from build123d import *

# Parameters (mm, degrees)
SKETCH1_W           = 57.02
SKETCH1_H           = 36.2
SKETCH1_R           = 2.2
BOSS_EXTRUDE1_DEPTH = 4
SKETCH2_W           = 57.02
SKETCH2_H           = 4
BOSS_EXTRUDE2_DEPTH = 29.05
SKETCH3_W           = 4
SKETCH3_H           = 42.02
BOSS_EXTRUDE3_DEPTH = 26
SKETCH5_R           = 7
CUT_EXTRUDE1_DEPTH  = 4
SKETCH6_W           = 42.02
SKETCH6_H           = 30
BOSS_EXTRUDE4_DEPTH = 2.5
SKETCH7_W           = 16
SKETCH7_H           = 16
CUT_EXTRUDE2_DEPTH  = 6.5


with BuildPart() as part:
    # Sketch1 → Boss-Extrude1 (new body)
    with BuildSketch(Plane(origin=(0, 0, 0), x_dir=(0, 0, -1), z_dir=(1, 0, 0))):
        Rectangle(SKETCH1_W, SKETCH1_H)
        with Locations((-24.51, -4.25)):
            Circle(SKETCH1_R, mode=Mode.SUBTRACT)
        with Locations((-24.51, -14.1)):
            Circle(SKETCH1_R, mode=Mode.SUBTRACT)
        with Locations((24.51, -4.25)):
            Circle(SKETCH1_R, mode=Mode.SUBTRACT)
        with Locations((24.51, -14.1)):
            Circle(SKETCH1_R, mode=Mode.SUBTRACT)
    extrude(amount=BOSS_EXTRUDE1_DEPTH)

    # Sketch2 → Boss-Extrude2 (add)
    with BuildSketch(Plane(origin=(4, 0, 0), x_dir=(0, 0, -1), z_dir=(1, 0, 0))):
        with Locations((0, 16.1)):
            Rectangle(SKETCH2_W, SKETCH2_H)
    extrude(amount=BOSS_EXTRUDE2_DEPTH)

    # Sketch3 → Boss-Extrude3 (add)
    with BuildSketch(Plane.XZ.offset(-14.1)):
        with Locations((31.05, 7.5)):
            Rectangle(SKETCH3_W, SKETCH3_H)
    extrude(amount=BOSS_EXTRUDE3_DEPTH)

    # Sketch5 → Cut-Extrude1 (cut)
    with BuildSketch(Plane(origin=(0, 18.1, 0), x_dir=(1, 0, 0), z_dir=(0, 1, 0))):
        with Locations((19, -10.79)):
            Circle(SKETCH5_R)
    extrude(amount=-CUT_EXTRUDE1_DEPTH, mode=Mode.SUBTRACT)

    # Sketch6 → Boss-Extrude4 (add)
    with BuildSketch(Plane(origin=(33.05, 0, 0), x_dir=(0, 0, -1), z_dir=(1, 0, 0))):
        with Locations((-7.5, 3.1)):
            Rectangle(SKETCH6_W, SKETCH6_H)
    extrude(amount=BOSS_EXTRUDE4_DEPTH)

    # Sketch7 → Cut-Extrude2 (cut)
    with BuildSketch(Plane(origin=(35.55, 0, 0), x_dir=(0, 0, -1), z_dir=(1, 0, 0))):
        with Locations((-7.51, 8.1)):
            Rectangle(SKETCH7_W, SKETCH7_H)
    extrude(amount=-CUT_EXTRUDE2_DEPTH, mode=Mode.SUBTRACT)


solid = part.part
For this review, take the finished solid that the model builds, in its own axes (mm). A direction names the side the tool comes from. Round coordinates to 2 decimals unless told otherwise and drop trailing zeros. Write each loop counter-clockwise with the first axis right and the second up, starting at its lowest first coordinate (ties: lowest second). Pieces come first, ordered by that corner, then holes. Notation, with made-up numbers: (-31.75, -36) -> (12.25, -36) arc R12 cw to (12.25, -13) -> close; hole circle Ø5 at (-17, 88.5). An arc over 180 degrees is marked (long way). Put each result on its own line as item: value.
Q1. Clearance check with flat-ended pins moving along their axes: pin 1 Ø1.5 at (y, z) = (1, -17.5) entering from +X; pin 2 Ø3 at (x, z) = (32, 9.5) entering from -Y; pin 3 Ø1 at (x, y) = (29.5, 5.5) entering from -Z; pin 4 Ø8.5 at (x, z) = (19, 8.5) entering from -Y. State where each tip first meets the part, or that it passes through.
Determined:
pin 1: stops at x = 4
pin 2: stops at y = -11.9
pin 3: stops at z = -13.51
pin 4: passes through
Q2. To check wall thickness, follow L1, parallel to Z at x = 3, y = -4; L2, parallel to Y at x = 1.85, z = 24.51; L3, parallel to Z at x = 32, y = 9. State the ranges of each line that lie inside material, in increasing order. Write a range as [from, to].
Determined:
L1: z = [-28.51, -26.7], [-22.32, 22.32], [26.7, 28.51]
L2: y = [-18.1, -16.3], [-11.9, -6.45], [-2.05, 18.1]
L3: z = [-13.51, -0.49], [15.51, 28.51]
Q3. Machinability: for faces 1 (the flat face through (33.05, 16, -21)), 2 (the flat face through (32, -11.9, 8)), 3 (the flat face through (32, 8, -0.49)), which of the approach directions +Z, -Z, +X, -X, +Y, -Y give a long, thin tool a straight path to every point of the face, cutting with its end or side? Answer none if there is none.
Determined:
face 1: -Z, +X, +Y, -Y
face 2: +Z, -Z, +X, -Y
face 3: +X
Q4. Consider section A-A on z = 1. State the section outline as (x, y) points.
Determined:
outline: (0, -18.1) -> (4, -18.1) -> (4, 14.1) -> (29.05, 14.1) -> (29.05, 16.1) -> (35.55, 16.1) -> (35.55, 18.1) -> (0, 18.1) -> close; (29.05, -11.9) -> (35.55, -11.9) -> (35.55, 0.1) -> (29.05, 0.1) -> close
Q5. Consider section B-B on y = 4.5. State the section outline as (x, z) points.
Determined:
outline: (0, -28.51) -> (4, -28.51) -> (4, 28.51) -> (0, 28.51) -> close; (29.05, -13.51) -> (35.55, -13.51) -> (35.55, -0.49) -> (29.05, -0.49) -> close; (29.05, 15.51) -> (35.55, 15.51) -> (35.55, 28.51) -> (29.05, 28.51) -> close
Q6. The part is to be moulded in two halves that separate along X. For faces 4 (the flat face through (29.05, -2, 7)), 5 (the flat face through (35.55, -3, 8)), 6 (the cylindrical face through (1.97, -3.59, -26.61)), 7 (the flat face through (4, -2, 0)), say which applies: released by +X, released by -X, zero draft, split by the parting line, or undercut.
Determined:
face 4: undercut
face 5: released by +X
face 6: zero draft
face 7: undercut
Q7. Consider section C-C on z = -24.51. State the section outline as (x, y) points, and give its area (3 significant figures).
Determined:
outline: (0, -18.1) -> (4, -18.1) -> (4, -16.3) -> (0, -16.3) -> close; (0, -11.9) -> (4, -11.9) -> (4, -6.45) -> (0, -6.45) -> close; (0, -2.05) -> (4, -2.05) -> (4, 14.1) -> (33.05, 14.1) -> (33.05, 18.1) -> (0, 18.1) -> close
area: 226 mm^2
Q8. Consider section D-D on y = -9.5. State the section outline as (x, z) points, and give its area (3 significant figures).
Determined:
outline: (0, -28.51) -> (4, -28.51) -> (4, 28.51) -> (0, 28.51) -> close; (29.05, -13.51) -> (35.55, -13.51) -> (35.55, 28.51) -> (29.05, 28.51) -> close
area: 501 mm^2
